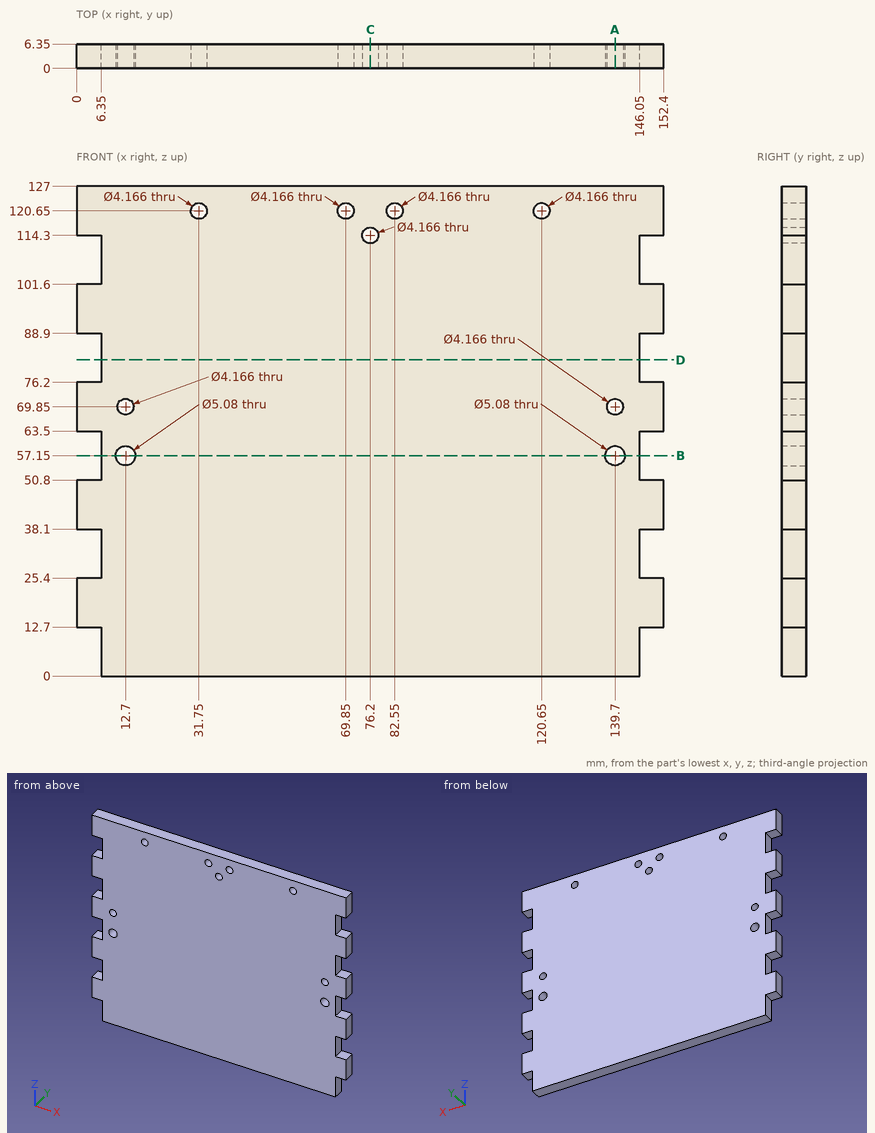
Answer from the drawing. Dimensions are ordinates in mm from the lowest x, y and z of the part. Round coordinates to 2 decimals unless told otherwise and drop trailing zeros. Write each loop counter-clockwise with the first axis right and the second up, starting at its lowest first coordinate (ties: lowest second). Pieces come first, ordered by that corner, then holes. Notation, with made-up numbers: (56, -25) - (112, -25) arc R11 cw to (112, -16) - close; hole circle Ø1 at (-16.75, 61.25). An arc over 180 degrees is marked (long way). Use a Markdown table: item, result.
(1) Straight lines are drawn through the part: line 1 along X through (y, z) = (3, 120.65); line 2 along X through (y, z) = (2.25, 57.15); line 3 along X through (y, z) = (1.25, 68.5) (1 decimal). For each, find the intervals that lie inside material, in ascending order. Write a range as [from, to].
Reported:
| item | result |
|---|---|
| line 1 | [0, 29.67], [33.83, 67.77], [71.93, 80.47], [84.63, 118.57], [122.73, 152.4] |
| line 2 | [6.35, 10.16], [15.24, 137.16], [142.24, 146.05] |
| line 3 | [0, 11.1], [14.3, 138.1], [141.3, 152.4] |
(2) Each of these flat-tipped pins is pushed along its axis until it touches: pin 1 Ø3 at (x, y) = (149, 2) entering from -Z; pin 2 Ø3 at (x, z) = (139.7, 57.15) entering from -Y. Where does it stop, or does it pass through?
Reported:
| item | result |
|---|---|
| pin 1 | z = 12.7 |
| pin 2 | through |
(3) The part is cut by section B-B (z = 57.15). Write down the section's boundary in (x, y).
Reported:
| item | result |
|---|---|
| outline | (6.35, 0) - (10.16, 0) - (10.16, 6.35) - (6.35, 6.35) - close; (15.24, 0) - (137.16, 0) - (137.16, 6.35) - (15.24, 6.35) - close; (142.24, 0) - (146.05, 0) - (146.05, 6.35) - (142.24, 6.35) - close |
(4) The part is cut by section C-C (x = 76.2). Write down the section's boundary in (y, z).
Reported:
| item | result |
|---|---|
| outline | (0, 0) - (6.35, 0) - (6.35, 112.22) - (0, 112.22) - close; (0, 116.38) - (6.35, 116.38) - (6.35, 127) - (0, 127) - close |
(5) The part is cut by section A-A (x = 139.7). Write down the section's boundary in (y, z).
Reported:
| item | result |
|---|---|
| outline | (0, 0) - (6.35, 0) - (6.35, 54.61) - (0, 54.61) - close; (0, 59.69) - (6.35, 59.69) - (6.35, 67.77) - (0, 67.77) - close; (0, 71.93) - (6.35, 71.93) - (6.35, 127) - (0, 127) - close |
(6) The part is cut by section D-D (z = 82). Write down the section's boundary in (x, y).
Reported:
| item | result |
|---|---|
| outline | (6.35, 0) - (146.05, 0) - (146.05, 6.35) - (6.35, 6.35) - close |
